For this review, take the finished solid that the model builds, in its own axes (mm). A direction names the side the tool comes from. Round coordinates to 2 decimals unless told otherwise and drop trailing zeros. Loops run counter-clockwise (first coordinate to the right, second up) from the corner with the lowest first, then second, coordinate; pieces in that order, holes last. Notation, with made-up numbers: (53, 68.25) -> (99, 68.25) arc R8 ccw to (99, 79.25) -> close; hole circle Ø6 at (78.5, 71). An arc over 180 degrees is marked (long way). Write each question's results on one line, items separated by ' | '.
```python
from build123d import *

# Parameters (mm, degrees)
SKETCH1_W           = 80
SKETCH1_H           = 80
SKETCH1_W_2         = 9
SKETCH1_H_2         = 43.113686922
BOSS_EXTRUDE1_DEPTH = 3
SKETCH3_W           = 8.2
SKETCH3_H           = 3.2
SKETCH3_W_2         = 3.2
SKETCH3_H_2         = 8.2
SKETCH3_W_3         = 20.2
SKETCH3_H_3         = 20.2
SKETCH3_H_4         = 5.2
CUT_EXTRUDE1_DEPTH  = 4
FILLET1_R           = 5
SKETCH4_W           = 5
SKETCH4_H           = 43.113686922
CUT_EXTRUDE2_DEPTH  = 4
FILLET2_R           = 7


with BuildPart() as part:
    # Sketch1 → Boss-Extrude1 (new body)
    with BuildSketch(Plane(origin=(0, 0, 0), x_dir=(1, 0, 0), z_dir=(0, 1, 0))):
        with Locations((40, 40)):
            Rectangle(SKETCH1_W, SKETCH1_H)
        with Locations((43.8, 37.4)):
            Rectangle(SKETCH1_W_2, SKETCH1_H_2, mode=Mode.SUBTRACT)
    extrude(amount=-BOSS_EXTRUDE1_DEPTH)

    # Sketch3 → Cut-Extrude1 (cut, through all)
    with BuildSketch(Plane(origin=(0, 0, 0), x_dir=(1, 0, 0), z_dir=(0, 1, 0))):
        with Locations((32, 1.5)):
            Rectangle(SKETCH3_W, SKETCH3_H)
        with Locations((78.5, 32)):
            Rectangle(SKETCH3_W_2, SKETCH3_H_2)
        with Locations((48, 1.5)):
            Rectangle(SKETCH3_W, SKETCH3_H)
        with Locations((1.5, 32)):
            Rectangle(SKETCH3_W_2, SKETCH3_H_2)
        with Locations((10, 10)):
            Rectangle(SKETCH3_W_3, SKETCH3_H_3)
        with Locations((70, 10)):
            Rectangle(SKETCH3_W_3, SKETCH3_H_3)
        with Locations((32, 78.5)):
            Rectangle(SKETCH3_W, SKETCH3_H)
        with Locations((1.5, 48)):
            Rectangle(SKETCH3_W_2, SKETCH3_H_2)
        with Locations((10, 70)):
            Rectangle(SKETCH3_W_3, SKETCH3_H_3)
        with Locations((78.5, 48)):
            Rectangle(SKETCH3_W_2, SKETCH3_H_2)
        with Locations((70, 70)):
            Rectangle(SKETCH3_W_3, SKETCH3_H_3)
        with Locations((48, 78.5)):
            Rectangle(SKETCH3_W, SKETCH3_H)
        with Locations((28.5, 14.85)):
            Rectangle(SKETCH3_W_2, SKETCH3_H_4)
        with Locations((28.5, 24.85)):
            Rectangle(SKETCH3_W_2, SKETCH3_H_4)
        with Locations((28.5, 70.85)):
            Rectangle(SKETCH3_W_2, SKETCH3_H_4)
    extrude(amount=-CUT_EXTRUDE1_DEPTH, mode=Mode.SUBTRACT)

    # Fillet1
    fillet1_edges = [part.edges().sort_by_distance(p)[0] for p in [
        (20.1, -1.5, -20.1),
        (59.9, -1.5, -20.1),
        (20.1, -1.5, -59.9),
        (59.9, -1.5, -59.9),
    ]]
    fillet(fillet1_edges, radius=FILLET1_R)

    # Sketch4 → Cut-Extrude2 (cut, through all)
    with BuildSketch(Plane(origin=(0, 0, 0), x_dir=(1, 0, 0), z_dir=(0, 1, 0))):
        with Locations((50.8, 37.4)):
            Rectangle(SKETCH4_W, SKETCH4_H)
    extrude(amount=-CUT_EXTRUDE2_DEPTH, mode=Mode.SUBTRACT)

    # Fillet2
    fillet2_edges = [part.edges().sort_by_distance(p)[0] for p in [
        (53.3, -1.5, -58.956843461),
        (53.3, -1.5, -15.843156539),
    ]]
    fillet(fillet2_edges, radius=FILLET2_R)


solid = part.part
```
1. Consider section C-C (x = 70). State the section outline as (y, z) points, plus the area to 3 significant figures.
Values found:
outline: (-3, -59.9) -> (0, -59.9) -> (0, -20.1) -> (-3, -20.1) -> close | area: 119 mm2
2. For pin 1 (1.5 mm diameter, centred on x = 67.5, y = -2, fed in from -Z); pin 2 (1 mm diameter, centred on x = 32, y = -2, fed in from -Z); pin 3 (1.5 mm diameter, centred on y = -1.5, z = -34, fed in from -X), all flat-tipped, find the tip position at first contact; note any pin that passes through.
Values found:
pin 1: stops at z = -59.9 | pin 2: stops at z = -76.9 | pin 3: stops at x = 3.1
3. Tool access review of faces 4 (the face through (3.1, -1, -48)), 5 (the face through (72, -1, -20.1)), 6 (the face through (28, -1, -68.25)): name each direction out of +Z, -Z, +X, -X, +Y, -Y from which nothing blocks a thin tool from reaching the whole face with its end or side.
Values found:
face 4: -X, +Y, -Y | face 5: +Z, +X, +Y, -Y | face 6: +Y, -Y
4. Consider section B-B (z = -40.5). State the section outline as (x, y) points, plus the area to 3 significant figures.
Values found:
outline: (0, -3) -> (39.3, -3) -> (39.3, 0) -> (0, 0) -> close; (53.3, -3) -> (80, -3) -> (80, 0) -> (53.3, 0) -> close | area: 198 mm2
5. To check wall thickness, follow probe 1 along Z at (x, y) = (29.5, -2.25); probe 2 along Z at (x, y) = (27, -1.95); probe 3 along X at (y, z) = (-0.35, -37). State the ranges of each line that lie inside material, in increasing order.
Values found:
probe 1: z = -76.9 to -73.45, -68.25 to -27.45, -22.25 to -17.45, -12.25 to -3.1 | probe 2: z = -80 to -73.45, -68.25 to -27.45, -22.25 to -17.45, -12.25 to 0 | probe 3: x = 0 to 39.3, 53.3 to 80
6. Consider section D-D (y = -2.5). Give the number of separate pieces and of enclosed holes in the cut face, plus the area to 3 significant figures.
Values found:
separate pieces: 1 | enclosed holes: 4 | area: 3,970 mm2
7. Draft analysis for pull direction Z (two halves, no side actions). For faces 1 (the face through (53.3, -1, -37)), 2 (the face through (52.1, -1, -2)), 3 (the face through (40, -1, 0)), state which applies: released by +Z, released by -Z, zero draft, split by the parting line, or undercut.
Values found:
face 1: undercut | face 2: zero draft | face 3: released by +Z
8. Consider section A-A (z = -71). State the section outline as (x, y) points, plus the area to 3 significant figures.
Values found:
outline: (20.1, -3) -> (26.9, -3) -> (26.9, 0) -> (20.1, 0) -> close; (30.1, -3) -> (59.9, -3) -> (59.9, 0) -> (30.1, 0) -> close | area: 110 mm2
